```python
from build123d import *

# Parameters (mm, degrees)
SKETCH3_W           = 1.016
SKETCH3_H           = 40.48125
CUT_EXTRUDE1_DEPTH  = 68.06130649
CUT_EXTRUDE2_REACH  = 69.061
SKETCH4_R           = 3.175
CIRPATTERN1_COUNT   = 3
SKETCH16_W          = 6.35
SKETCH16_H          = 6.35
CUT_EXTRUDE7_DEPTH  = 68.06130649
SKETCH24_R          = 16.335149264
CUT_EXTRUDE13_DEPTH = 68.06130649
SKETCH25_W          = 2.685482999
SKETCH25_H          = 26.348135083
CUT_EXTRUDE14_DEPTH = 68.06130649


# Read off the part's stored shape, not the designer's step: Cut-Extrude3, Cut-Extrude4
with BuildPart() as part:
    # Sketch1 → Revolve1 (revolve)
    with BuildSketch(Plane(origin=(0, 0, 0), x_dir=(0, 0, -1), z_dir=(1, 0, 0)), mode=Mode.PRIVATE) as revolve1_sk:
        Polygon((34.925, -27.1795875), (15.875, -27.7749), (15.875, -26.98115), (12.7, -26.98115), (12.7, -39.97325), (12.192, -40.48125), (0.508, -40.48125), (0, -39.97325), (0, -15.875), (34.925, -15.875), align=None)
    revolve(revolve1_sk.sketch.rotate(Axis((0, 0, 0), (0, 0, -1)), 270), axis=Axis((0, 0, 0), (0, 0, -1)))

    # Sketch3 → Cut-Extrude1 (cut, through all)
    with BuildSketch(Plane.XY):
        with Locations((0, -20.240625)):
            Rectangle(SKETCH3_W, SKETCH3_H)
    extrude(amount=-CUT_EXTRUDE1_DEPTH, mode=Mode.SUBTRACT)

    # Sketch4 → Cut-Extrude2 (cut, up to next)
    with BuildSketch(Plane.XY, mode=Mode.PRIVATE) as cut_extrude2_sk1:
        with Locations((34.13125, 0)):
            Circle(SKETCH4_R)
    cut_extrude2_tool1 = extrude(cut_extrude2_sk1.sketch, amount=-CUT_EXTRUDE2_REACH, mode=Mode.PRIVATE) & part.part
    # Sketch4 → Cut-Extrude2 (cut, up to next)
    with BuildSketch(Plane.XY, mode=Mode.PRIVATE) as cut_extrude2_sk2:
        with Locations((-34.13125, 0)):
            Circle(SKETCH4_R)
    cut_extrude2_tool2 = extrude(cut_extrude2_sk2.sketch, amount=-CUT_EXTRUDE2_REACH, mode=Mode.PRIVATE) & part.part
    cut_extrude2_1 = cut_extrude2_tool1.solids().sort_by_distance((34.13125, 0, 0))[0]
    add(cut_extrude2_1, mode=Mode.SUBTRACT)
    cut_extrude2_2 = cut_extrude2_tool2.solids().sort_by_distance((-34.13125, 0, 0))[0]
    add(cut_extrude2_2, mode=Mode.SUBTRACT)
    cut_extrude2 = cut_extrude2_1 + cut_extrude2_2  # Cut-Extrude2 as one shape, for the pattern or mirror that repeats it

    # Cut-Extrude3 outline → Cut-Extrude3 (revolve, cut)
    with BuildSketch(Plane(origin=(34.13125, 0, 0), x_dir=(1, 0, 0), z_dir=(0, -1, 0))):
        Polygon((3.175, 0), (3.175, -0.137481533), (3.312481533, 0), align=None)
    cut_extrude3 = revolve(axis=Axis((34.13125, 0, 0), (0, 0, 1)), mode=Mode.SUBTRACT)

    # Cut-Extrude4 outline → Cut-Extrude4 (revolve, cut)
    with BuildSketch(Plane(origin=(34.13125, 0, 0), x_dir=(1, 0, 0), z_dir=(0, -1, 0))):
        Polygon((3.312481533, -12.7), (3.175, -12.562518467), (3.175, -12.7), align=None)
    cut_extrude4 = revolve(axis=Axis((34.13125, 0, 0), (0, 0, 1)), mode=Mode.SUBTRACT)

    # CirPattern1: Cut-Extrude2, Cut-Extrude3, Cut-Extrude4 ×3 about axis
    cirpattern1_axis = Axis((0, 0, 0), (0, 0, 1))
    add([cut_extrude2.rotate(cirpattern1_axis, i * 360 / CIRPATTERN1_COUNT) for i in range(1, CIRPATTERN1_COUNT)], mode=Mode.SUBTRACT)
    add([cut_extrude3.rotate(cirpattern1_axis, i * 360 / CIRPATTERN1_COUNT) for i in range(1, CIRPATTERN1_COUNT)], mode=Mode.SUBTRACT)
    add([cut_extrude4.rotate(cirpattern1_axis, i * 360 / CIRPATTERN1_COUNT) for i in range(1, CIRPATTERN1_COUNT)], mode=Mode.SUBTRACT)

    # Sketch16 → Cut-Extrude7 (cut, through all)
    with BuildSketch(Plane.XY):
        with Locations((0, 15.875)):
            Rectangle(SKETCH16_W, SKETCH16_H)
    extrude(amount=-CUT_EXTRUDE7_DEPTH, mode=Mode.SUBTRACT)

    # Sketch24 → Cut-Extrude13 (cut, through all)
    with BuildSketch(Plane.XY):
        Circle(SKETCH24_R)
    extrude(amount=-CUT_EXTRUDE13_DEPTH, mode=Mode.SUBTRACT)

    # Sketch25 → Cut-Extrude14 (cut, through all)
    with BuildSketch(Plane.XY):
        with Locations((0.025334746, -28.373320916)):
            Rectangle(SKETCH25_W, SKETCH25_H)
    extrude(amount=-CUT_EXTRUDE14_DEPTH, mode=Mode.SUBTRACT)


solid = part.part
```
The listing builds one solid part. Answer for the finished solid, in the listing's coordinates (mm). A direction names the side the tool comes from. Give positions to 0.01 mm unless a question says otherwise; leave off trailing zeros. Write each loop counter-clockwise with the first axis right and the second up, starting at its lowest first coordinate (ties: lowest second). Pieces come first, ordered by that corner, then holes. Notation, with made-up numbers: (72, 6.5) - (115, 6.5) arc R10 ccw to (115, 20.5) - close; hole circle Ø3 at (84, 34.25). An arc over 180 degrees is marked (long way). Use one line per item in the form item = value. Start each with the question number.
1) A tool of negligible diameter and unlimited length cuts with its end or side. For faces 4 (the face through (1.368, -26, -13)), 5 (the face through (-23, -15, -15.875)), 6 (the face through (-16.324, -0.61, -17.218)), from which of +Z, -Z, +X, -X, +Y, -Y can it reach the whole face along a straight path? Write none if from no direction.
2) Find section C-C on z = -4. Count the separate pieces of the cut face and the enclosed holes in it, plus the area to 3 significant figures.
3) Flat-ended cylindrical pins translate along their axes: pin 1 Ø5 at (x, y) = (17.07, -29.56) entering from +Z; pin 2 Ø10 at (y, z) = (-20, -30.5) entering from -X; pin 3 Ø1.9 at (x, z) = (1.5, -17.5) entering from -Y; pin 4 Ø1 at (y, z) = (7.5, -17.5) entering from +X. Find the tip coordinate at first contact, or state that the pin passes through.
4) Find section A-A on x = 0. Determine the outline of the cut face in (y, z) (3 decimals).
5) Find section B-B on z = -33. Determine the outline of the cut face in (x, y) (3 decimals).
6) Consider line 1 along Y through (x, z) = (-15, -2.5); line 2 along Z through (x, y) = (-8, 27); line 3 along X through (y, z) = (2.5, -1.5). Determine where each line is inside the solid, lowest interval first. Write a range as from..to.
7) The mould has two halves that part along Y. Classify faces 1 (the face through (17, -1, 0)), 2 (the face through (-3.175, 18, -17)), 3 (the face through (16.29, -1.24, -17.22)): pulls with the +Y half, pulls with the -Y half, needs draft (parallel to the pull), parting line crosses it, or undercut.
Geometry results:
q1.face_4 = +Z, -Z, -Y
q1.face_5 = none
q1.face_6 = +Z, -Z
q2.separate_pieces = 1
q2.enclosed_holes = 6
q2.area = 4,040 mm2
q3.pin_1 = through
q3.pin_2 = -22.84
q3.pin_3 = -27.72
q3.pin_4 = 26.83
q4.outline = (19.05, -34.925) - (27.18, -34.925) - (27.775, -15.875) - (26.981, -15.875) - (26.981, -12.7) - (39.973, -12.7) - (40.481, -12.192) - (40.481, -0.508) - (39.973, 0) - (19.05, 0) - close
q5.outline = (-3.175, 16.024) - (-3.175, 19.05) - (3.175, 19.05) - (3.175, 16.024) arc R16.335 cw to (1.368, -16.278) - (1.368, -27.205) arc R27.24 ccw (long way) to (-1.317, -27.208) - (-1.317, -16.282) arc R16.335 cw to start
q6.line_1 = -37.6..-31.97, -27.15..-6.47, 6.47..27.15, 31.97..37.6
q6.line_2 = -12.7..0
q6.line_3 = -40.4..-36.09, -32.17..-16.14, 16.14..32.17, 36.09..40.4
q7.face_1 = needs draft
q7.face_2 = undercut
q7.face_3 = undercut
